The figure shows three views and two pictorial views of one solid part (mm, origin at its lowest corner). Answer the questions. A direction names the side the tool comes from. Round coordinates to 2 decimals unless told otherwise and drop trailing zeros. Order: outer loops, then holes, each group sorted by start corner. A loop starts at its lowest first (then second) coordinate and runs counter-clockwise, first axis right, second up.
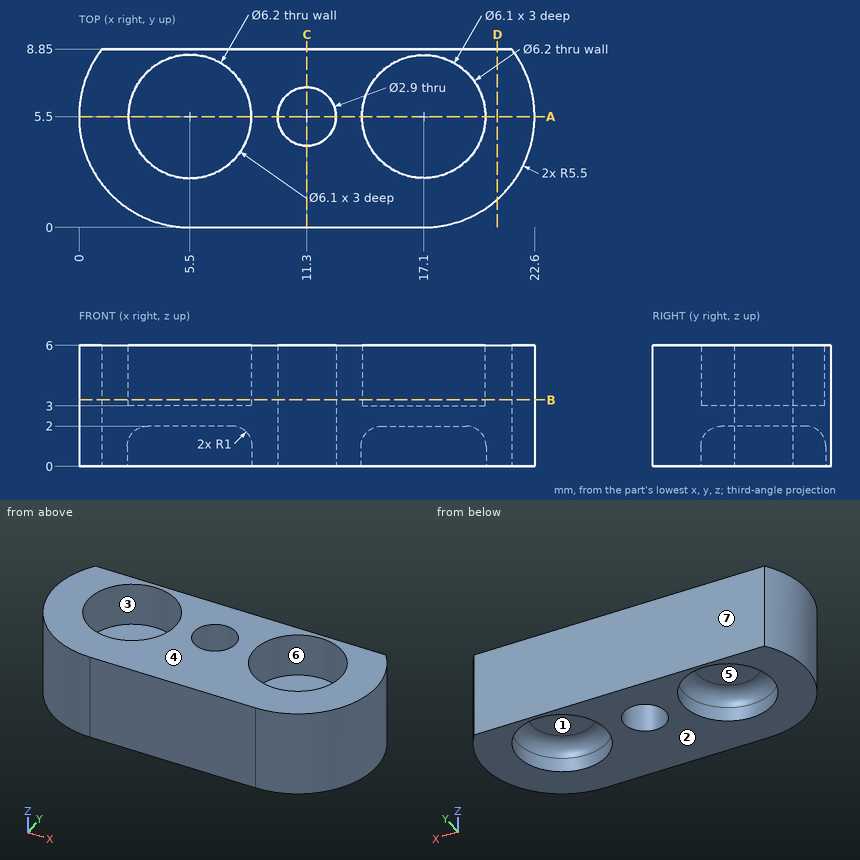
Item 1: Find section D-D (x = 20.75). Write down the section's boundary in (y, z).
Item 2: For a pull along Y with two mould halves and no side action, classify the marked faces 4, 5, 6 and 7 as released by +Y, released by -Y, zero draft, split by the parting line, or undercut.
Item 3: Find the intervals of material crossed by line 1 along Y through (x, z) = (17.1, 3.7); line 2 along X through (y, z) = (8, 5.85); line 3 along X through (y, z) = (7.5, 3.7), in increasing order.
Item 4: A tool of negligible diameter and unlimited length cuts with its end or side. For the marked faces 1, 2 and 3, from which of +Z, -Z, +X, -X, +Y, -Y can it reach the whole face along a straight path? Write none if from no direction.
Item 5: Given pin 1 (1 mm diameter, centred on x = 16, y = 6, fed in from -Z); pin 2 (5 mm diameter, centred on x = 5.5, y = 5.5, fed in from +Z), each flat-ended and moving along its own axis, determine where each tip first touches the part or whether it passes through.
Item 6: Find section A-A (y = 5.5). Write down the section's boundary in (x, z), plus the area to 3 significant figures.
Item 7: Find section B-B (z = 3.3). Write down the section's boundary in (x, y).
Item 8: Find section C-C (x = 11.3). Write down the section's boundary in (y, z), plus the area to 3 significant figures.
Model answer:
1. outline: (1.39, 0) - (8.85, 0) - (8.85, 6) - (1.39, 6) - close
2. face 4: zero draft
2. face 5: undercut
2. face 6: undercut
2. face 7: released by +Y
3. line 1: y = 0 to 2.45, 8.55 to 8.85
3. line 2: x = 0.6 to 3.75, 7.25 to 15.35, 18.85 to 22
3. line 3: x = 0.38 to 3.2, 7.8 to 14.8, 19.4 to 22.22
4. face 1: -Z
4. face 2: -Z, +X, -X, +Y, -Y
4. face 3: +Z
5. pin 1: stops at z = 2
5. pin 2: stops at z = 3
6. outline: (0, 0) - (2.4, 0) - (2.4, 1) arc R1 cw to (3.4, 2) - (7.6, 2) arc R1 cw to (8.6, 1) - (8.6, 0) - (9.85, 0) - (9.85, 6) - (8.55, 6) - (8.55, 3) - (2.45, 3) - (2.45, 6) - (0, 6) - close; (12.75, 0) - (14, 0) - (14, 1) arc R1 cw to (15, 2) - (19.2, 2) arc R1 cw to (20.2, 1) - (20.2, 0) - (22.6, 0) - (22.6, 6) - (20.15, 6) - (20.15, 3) - (14.05, 3) - (14.05, 6) - (12.75, 6) - close
6. area: 57.7 mm2
7. outline: (1.14, 8.85) arc R5.5 ccw to (5.5, 0) - (17.1, 0) arc R5.5 ccw to (21.46, 8.85) - close; hole circle Ø6.1 at (5.5, 5.5); hole circle Ø2.9 at (11.3, 5.5); hole circle Ø6.1 at (17.1, 5.5)
8. outline: (0, 0) - (4.05, 0) - (4.05, 6) - (0, 6) - close; (6.95, 0) - (8.85, 0) - (8.85, 6) - (6.95, 6) - close
8. area: 35.7 mm2
